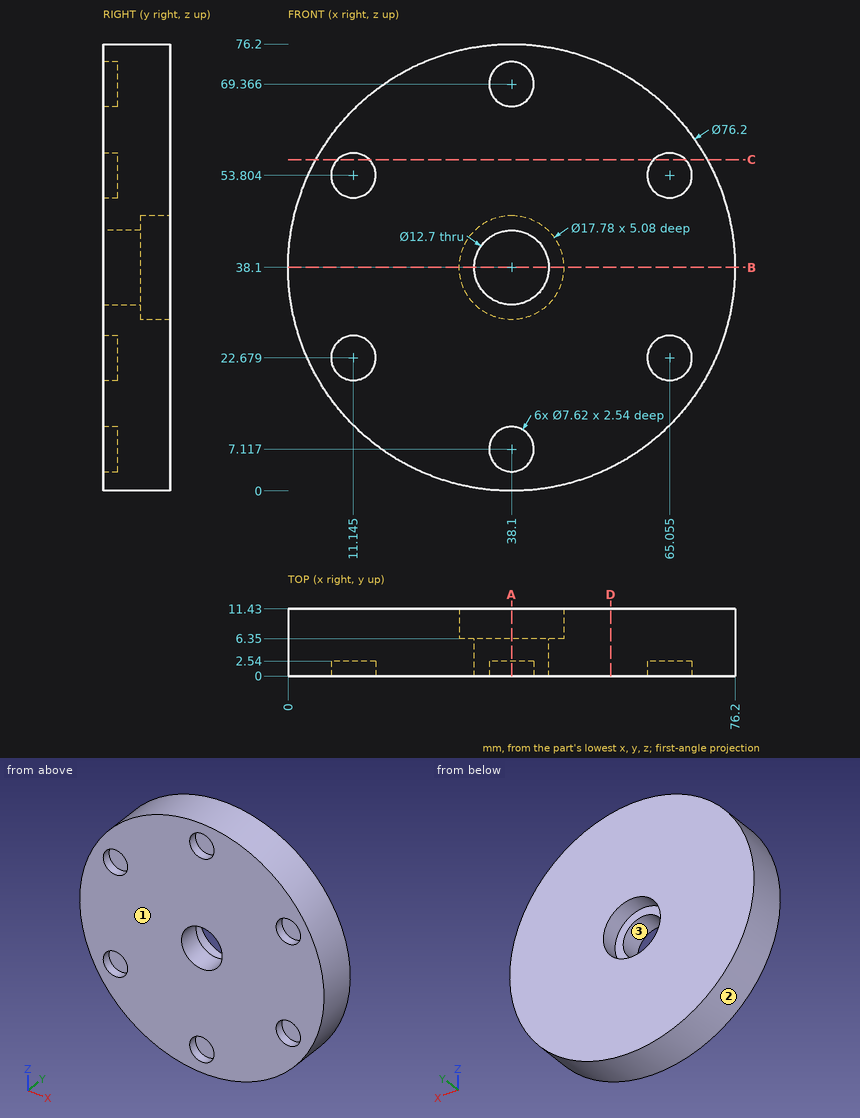
Check sheet for the drawn part. Datum: minimum x, y, z corner. Units: mm. Coordinates: 2 decimals unless noted, no trailing zeros. Loops run counter-clockwise (first coordinate to the right, second up) from the corner with the lowest first, then second, coordinate; pieces in that order, holes last. Notation, with made-up numbers: (52.5, -14) -> (76.5, -14) arc R15 cw to (76.5, 5) -> close; hole circle Ø7 at (77, 62). An arc over 180 degrees is marked (long way). Answer as CSV lines item,"result".
1) Depth check by flat-ended pin: pin 1 (4.5 mm diameter, centred on x = 38.1, z = 7.12, fed in from -Y); pin 2 (1.5 mm diameter, centred on x = 68.5, y = 7, fed in from -Z) (1 decimal); pin 3 (14.5 mm diameter, centred on x = 38.1, z = 38.1, fed in from +Y). Enter the tip coordinate at first touch or a pass-through.
Found:
pin 1,"stops at y = 2.54"
pin 2,"stops at z = 14.2"
pin 3,"stops at y = 6.35"
2) Cross-section at D-D, the plane x = 55. Record the cut outline in (y, z).
Found:
outline,"(0, 3.95) -> (11.43, 3.95) -> (11.43, 72.25) -> (0, 72.25) -> close"
3) Release check for a two-part mould opening along Z. For the marked faces 1, 2 and 3 record: +Z half, -Z half, draft (parallel to the pull), parting line (faces both ways), or undercut.
Found:
face 1,"draft"
face 2,"parting line"
face 3,"undercut"
4) Cross-section at B-B, the plane z = 38.1. Record the cut outline in (x, y).
Found:
outline,"(0, 0) -> (31.75, 0) -> (31.75, 6.35) -> (29.21, 6.35) -> (29.21, 11.43) -> (0, 11.43) -> close; (44.45, 0) -> (76.2, 0) -> (76.2, 11.43) -> (46.99, 11.43) -> (46.99, 6.35) -> (44.45, 6.35) -> close"
5) Cross-section at A-A, the plane x = 38.1. Record the cut outline in (y, z).
Found:
outline,"(0, 0) -> (11.43, 0) -> (11.43, 29.21) -> (6.35, 29.21) -> (6.35, 31.75) -> (0, 31.75) -> (0, 10.93) -> (2.54, 10.93) -> (2.54, 3.31) -> (0, 3.31) -> close; (0, 44.45) -> (6.35, 44.45) -> (6.35, 46.99) -> (11.43, 46.99) -> (11.43, 76.2) -> (0, 76.2) -> (0, 73.18) -> (2.54, 73.18) -> (2.54, 65.56) -> (0, 65.56) -> close"
6) Cross-section at C-C, the plane z = 56.5. Record the cut outline in (x, y), then the cut area to 3 significant figures.
Found:
outline,"(4.74, 0) -> (8.45, 0) -> (8.45, 2.54) -> (13.84, 2.54) -> (13.84, 0) -> (62.36, 0) -> (62.36, 2.54) -> (67.75, 2.54) -> (67.75, 0) -> (71.46, 0) -> (71.46, 11.43) -> (4.74, 11.43) -> close"
area,"735 mm2"
7) Thickness scan on L1, parallel to X at y = 10, z = 38.5; L2, parallel to Z at x = 13.5, y = 2 (1 decimal); L3, parallel to X at y = 1, z = 4.5 (1 decimal). Record the ranges inside material, lowest first. Write a range as from..to.
Found:
L1,"x = 0..29.22, 46.98..76.2"
L2,"z = 9..19.7, 25.7..50.8, 56.8..67.2"
L3,"x = 20.1..35.3, 40.9..56.1"
